```python
from build123d import *

# Parameters (mm, degrees)
F1_DEPTH  = 14
F2_R      = 2.1
F3_DEPTH  = 25
F5_W      = 9
F5_H      = 3.5
F6_DEPTH  = 10
F4_R      = 2.1
F7_DEPTH  = 1.75
F8_R      = 1.625
F9_DEPTH  = 2.5
F10_DEPTH = 25
F11_R     = 2.85
F11_R_2   = 1.625
F12_DEPTH = 2


with BuildPart() as f1:
    # F0 (on Top) → F1 (new body)
    with BuildSketch(Plane.XY):
        Polygon((5, 0), (0, 0), (0, -19.5), (5, -24.5), (5, -39), (12.5, -39), (12.5, -24.5), (17.5, -19.5), (17.5, 0), (12.5, 0), (12.5, -17.5), (5, -17.5), align=None)
    extrude(amount=F1_DEPTH)

    # F2 (on face) → F3 (cut)
    with BuildSketch(Plane.XZ.offset(39)):
        with Locations((8.75, 7)):
            Circle(F2_R)
    extrude(amount=-F3_DEPTH, mode=Mode.SUBTRACT)

    # F5 (on face) → F6 (cut)
    with BuildSketch(Plane.XY.offset(14)):
        with Locations((8.75, -17.5)):
            Rectangle(F5_W, F5_H)
    extrude(amount=-F6_DEPTH, mode=Mode.SUBTRACT)

    # F4 (on face) → F7 (cut)
    with BuildSketch(Plane(origin=(0, -17.5, 0), x_dir=(-1, 0, 0), z_dir=(0, 1, 0))):
        Polygon((-5, 4.2150635095), (-5, 9.7849364905), (-8.75, 11.95), (-12.5, 9.7849364905), (-12.5, 4.2150635095), (-8.75, 2.05), align=None)
        with Locations((-8.75, 7)):
            Circle(F4_R, mode=Mode.SUBTRACT)
    extrude(amount=-F7_DEPTH, mode=Mode.SUBTRACT)

    # F8 (on face) → F9 (cut)
    with BuildSketch(Plane.YZ.offset(17.5)):
        Polygon((-2.1854174377, 5.375), (-2.1854174377, 8.625), (-5, 10.25), (-7.8145825623, 8.625), (-7.8145825623, 5.375), (-5, 3.75), align=None)
        with Locations((-5, 7)):
            Circle(F8_R, mode=Mode.SUBTRACT)
    extrude(amount=-F9_DEPTH, mode=Mode.SUBTRACT)

    # F10 (cut): a face of the model
    f10_faces = [f1.faces().sort_by_distance(p)[0] for p in [
        (17.5, -5, 7),
    ]]
    extrude(f10_faces, amount=-F10_DEPTH, mode=Mode.SUBTRACT)

    # F11 (on face) → F12 (cut)
    with BuildSketch(Plane(origin=(0, 0, 0), x_dir=(0, -1, 0), z_dir=(-1, 0, 0))):
        with Locations((5, 7)):
            Circle(F11_R)
        with Locations((5, 7)):
            Circle(F11_R_2, mode=Mode.SUBTRACT)
    extrude(amount=-F12_DEPTH, mode=Mode.SUBTRACT)


solid = f1.part
```
Geometry: final body of the model. Coordinates: model frame, mm. A direction names the side the tool comes from. Round coordinates to 2 decimals unless told otherwise and drop trailing zeros. Order: outer loops, then holes, each group sorted by start corner. A loop starts at its lowest first (then second) coordinate and runs counter-clockwise, first axis right, second up. Notation, with made-up numbers: M 70,-34.75 L 82,-34.75 A26 cw 82,-18.75 Z; hole C -35.75,-10 d4. An arc over 180 degrees is marked long. One line per item, written item: value.
(1) Cut plane C-C (y = -21.5). Return the cut outline in (x, z).
Result sheet:
outline: M 2,0 L 15.5,0 L 15.5,14 L 2,14 Z; hole C 8.75,7 d4.2
(2) Reachability of faces 1 (the flat face through (13.25, -18, 9)), 2 (the flat face through (12.5, -32, 7)), 3 (the flat face through (10.462, -18.363, 3.039)), 4 (the flat face through (15, -6.3, 5.6)), 5 (the flat face through (5, -9, 7)) from +Z, -Z, +X, -X, +Y, -Y: full face, straight path, thin tool, end or side. Return the list, or none.
Result sheet:
face 1: +Z
face 2: +Z, -Z, +X, -Y
face 3: +Z, +Y
face 4: +X
face 5: +Z, -Z, +Y
(3) Cut plane D-D (z = 7). Give the number of separate pieces and of enclosed holes in the cut face, and give its area (3 significant figures).
Result sheet:
separate pieces: 4
enclosed holes: 0
area: 237 mm2
(4) Pin query (flat end, axial travel): P1, Ø2, axis at y = -21, z = 8, coming from the +X side; P2, Ø3, axis at x = 7, z = 2.5, coming from the +Y side; P3, Ø5, axis at y = -27.5, z = 2, coming from the +X side; P4, Ø1.7, axis at y = -4.5, z = 7.5, coming from the -X side. Return the tip coordinate at first contact, or that it passes through.
Result sheet:
P1: x = 17
P2: y = -17.5
P3: x = 12.5
P4: through
(5) Line query: probe 1 along Z at (x, y) = (0.5, -5); probe 2 along Z at (x, y) = (8.75, -25.75); probe 3 along X at (y, z) = (-17, 3). Output: solid intervals per line, ascending. Write a range as [from, to].
Result sheet:
probe 1: [0, 4.15], [9.85, 14]
probe 2: [0, 4.9], [9.1, 14]
probe 3: [0, 5], [12.5, 17.5]
(6) Cut plane B-B (z = 12.25). Return the cut outline in (x, y).
Result sheet:
outline: M 0,-19.5 L 5,-24.5 L 5,-39 L 12.5,-39 L 12.5,-24.5 L 17.5,-19.5 L 17.5,0 L 12.5,0 L 12.5,-15.75 L 13.25,-15.75 L 13.25,-19.25 L 4.25,-19.25 L 4.25,-15.75 L 5,-15.75 L 5,0 L 0,0 Z
(7) Pull-direction query (Z, two-part tool) for faces 6 (the flat face through (12.5, -9, 7)), 7 (the flat face through (9, -19, 0)), 8 (the flat face through (16, -2.185, 7)); classes: pulls with the +Z half, pulls with the -Z half, needs draft (parallel to the pull), parting line crosses it, or undercut.
Result sheet:
face 6: needs draft
face 7: pulls with the -Z half
face 8: undercut
(8) Cut plane A-A (y = -14). Return the cut outline in (x, z), and give its area (3 significant figures).
Result sheet:
outline: M 0,0 L 5,0 L 5,14 L 0,14 Z; M 12.5,0 L 17.5,0 L 17.5,14 L 12.5,14 Z
area: 140 mm2
